For this review, take the finished solid that the model builds, in its own axes (mm). Face numbers are marked on the shaded views. A direction names the side the tool comes from. Give positions to 0.01 mm unless a question says otherwise; leave off trailing zeros. Answer in a Markdown table with one row per item.
```python
from build123d import *

# Parameters (mm, degrees)
F0_W        = 180
F0_H        = 80
F2_W        = 62
F2_H        = 62
F4_W        = 51
F4_H        = 51
F5_DEPTH    = 30
F6_T        = 5
F6_T3_DEPTH = 40
F6_T5_DEPTH = 61
F6_T7_DEPTH = 61
F7_R        = 5


# Not quite as in the source:
# - a shell that OpenCascade refuses in one call is made with other operations: the cavity is built on its own and cut out


with BuildPart() as f3:
    # F0 (on Top) → F3 section 0
    with BuildSketch(Plane.XY):
        Rectangle(F0_W, F0_H)
    # F2 (on offset) → F3 section 1
    with BuildSketch(Plane.XY.offset(40)):
        Rectangle(F2_W, F2_H)
    loft()

    # F4 (on face) → F5 (cut)
    with BuildSketch(Plane.XY.offset(40)):
        Rectangle(F4_W, F4_H)
    extrude(amount=-F5_DEPTH, mode=Mode.SUBTRACT)

    # F6: shell of thickness 5, made by hand


with BuildPart() as f6_core1:
    # F6_t2: copy of F3
    add(f3.part)

    # the walls: a layer under each face that stays
    f6_faces = [f6_core1.faces().sort_by_distance(p)[0] for p in [
        (0, 35.5, 20),
        (-60.5, 0, 20),
        (26.5714285714, 26.5714285714, 40),
        (60.5, 0, 20),
        (0, -35.5, 20),
        (-25.5, 0, 25),
        (0, 25.5, 25),
        (25.5, 0, 25),
        (0, -25.5, 25),
        (0, 0, 10),
    ]]
    thicken(f6_faces, amount=-F6_T, mode=Mode.SUBTRACT)

    # F6_s4 → F6_t3 (cut)
    with BuildSketch(Plane.XY.offset(5)):
        Polygon((-25.45, 25.45), (-30.5, 25.5), (-30.5, 30.5), (-25.5, 30.5), align=None)
        Polygon((-25.45, -25.45), (-30.5, -25.5), (-30.5, -30.5), (-25.5, -30.5), align=None)
        Polygon((25.45, 25.45), (25.5, 30.5), (30.5, 30.5), (30.5, 25.5), align=None)
        Polygon((25.45, -25.45), (30.5, -25.5), (30.5, -30.5), (25.5, -30.5), align=None)
    extrude(amount=F6_T3_DEPTH, mode=Mode.SUBTRACT)

    # F6_s6 → F6_t5 (cut)
    with BuildSketch(Plane.XZ.offset(-30.5)):
        Polygon((-25.45, 10.05), (-30.5, 10), (-30.5, 5), (-25.5, 5), align=None)
        Polygon((25.45, 10.05), (30.5, 10), (30.5, 5), (25.5, 5), align=None)
    extrude(amount=F6_T5_DEPTH, mode=Mode.SUBTRACT)

    # F6_s8 → F6_t7 (cut)
    with BuildSketch(Plane.YZ.offset(-30.5)):
        Polygon((25.45, 10.05), (30.5, 10), (30.5, 5), (25.5, 5), align=None)
        Polygon((-25.45, 10.05), (-30.5, 10), (-30.5, 5), (-25.5, 5), align=None)
    extrude(amount=F6_T7_DEPTH, mode=Mode.SUBTRACT)


with BuildPart() as f3_1:
    add(f3.part)

    # what is left inside the walls is the cavity
    f6_cavity = [f6_core1.part.solids().sort_by_distance(p)[0] for p in [
        (8.772982, -19.739209, 0.05),
    ]]
    add(f6_cavity, mode=Mode.SUBTRACT)

    # F7
    f7_edges = [f3_1.edges().sort_by_distance(p)[0] for p in [
        (60.5, -35.5, 20),
        (60.5, 35.5, 20),
        (-60.5, 35.5, 20),
        (-60.5, -35.5, 20),
    ]]
    fillet(f7_edges, radius=F7_R)


solid = f3_1.part
```
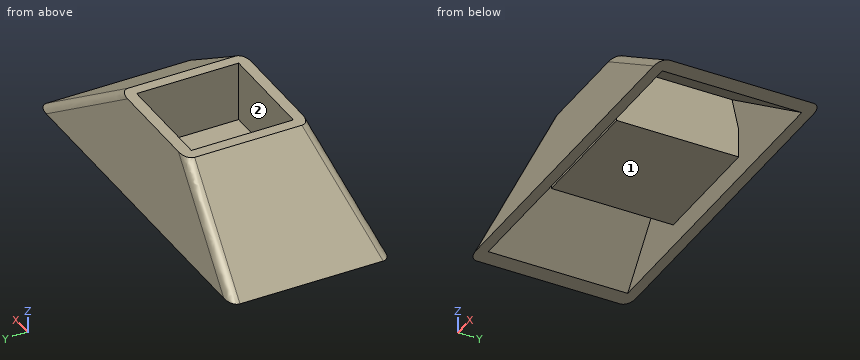
1. Wall thickness on line 1 (X direction, y = 7, z = 7.5); line 2 (X direction, y = 14, z = 26); line 3 (Y direction, x = -11.5, z = 17) (3 decimals): over which ranges is each line inside the solid? List them lowest first. Write a range as [from, to].
Values:
| item | result |
|---|---|
| line 1 | x = [-78.94, -70.03], [-30.5, 30.5], [70.03, 78.94] |
| line 2 | x = [-51.65, -42.74], [-30.5, -25.5], [25.5, 30.5], [42.74, 51.65] |
| line 3 | y = [-36.175, -31.05], [-30.5, -25.5], [25.5, 30.5], [31.05, 36.175] |
2. We need section A-A, the plane z = 7. Count the separate pieces of the cut face and the enclosed holes in it, and give its area (3 significant figures).
Values:
| item | result |
|---|---|
| separate pieces | 2 |
| enclosed holes | 1 |
| area | 6,520 mm^2 |
3. Clearance check with flat-ended pins moving along their axes: pin 1 (3 mm diameter, centred on x = 37.5, z = 11, fed in from +Y); pin 2 (12 mm diameter, centred on x = -10, z = 7, fed in from -Y) (3 decimals); pin 3 (15 mm diameter, centred on x = -11.5, z = 18.5, fed in from +Y) (3 decimals). State where each tip first meets the part, or that it passes through.
Values:
| item | result |
|---|---|
| pin 1 | stops at y = 37.86 |
| pin 2 | stops at y = -39.775 |
| pin 3 | stops at y = 37.525 |
4. For the marked faces 1 and 2, list the 3-axis set-ups (+Z, -Z, +X, -X, +Y, -Y) from which the entire face can be reached by the end or side of a thin tool; tool diameter is ignored.
Values:
| item | result |
|---|---|
| face 1 | -Z |
| face 2 | +Z |
